Build history of the part. All positions in model axes, mm. Face numbers are marked on the shaded views. Give positions to 0.01 mm unless a question says otherwise; leave off trailing zeros. Order: outer loops, then holes, each group sorted by start corner. A loop starts at its lowest first (then second) coordinate and runs counter-clockwise, first axis right, second up. Notation, with made-up numbers: (53.5, 1.5) - (58.5, 1.5) arc R18 cw to (58.5, 33.5) - close; hole circle Ø1 at (-11.75, -19). An arc over 180 degrees is marked (long way). Write each question's results on one line, items separated by ' | '. Start each with the question number.
1) Cut at A-A on z = 0. List the corners of the cut face in (x, y).
2) Drill centre lines: line 1 along X through (y, z) = (13.6, 0); line 2 along Y through (x, z) = (-67.5, -224.5); line 3 along X through (y, z) = (-13.05, -235). Where is each one in solid material? Low to high. Write a range as from..to.
3) Two-plate mould, pull along X, no slides. Class the marked faces 1, 2 and 3: +X half, -X half, draft (parallel to the pull), parting line (faces both ways), or undercut.
4) Cut at D-D on z = 145.5. List the corners of the cut face in (x, y).
5) Drop flat-ended pins along their axis: pin 1 Ø14 at (x, z) = (-203.52, 117.5) entering from +Y; pin 2 Ø6 at (y, z) = (13, -211) entering from -X; pin 3 Ø5 at (x, y) = (-31, 8.5) entering from -Z. Give the stop position or say it passes through.
6) Cut at C-C on x = 74.5. List the corners of the cut face in (y, z).
7) Cut at B-B on x = -235. List the corners of the cut face in (y, z).
from build123d import *

# Parameters (mm, degrees)
SKETCH1_R           = 260
SKETCH1_R_2         = 6
SKETCH1_R_3         = 219.5
BOSS_EXTRUDE1_DEPTH = 17
SKETCH2_R           = 250
CUT_EXTRUDE1_DEPTH  = 12
CUT_EXTRUDE2_DEPTH  = 370.264133108
BOSS_EXTRUDE2_DEPTH = 130


with BuildPart() as part:
    # Sketch1 → Boss-Extrude1 (new, symmetric)
    with BuildSketch(Plane(origin=(0, 0, 0), x_dir=(1, 0, 0), z_dir=(0, 1, 0))):
        with Locations(Location((0, 0, 0), (0, 0, 270))):
            Circle(SKETCH1_R)
        with Locations(Location((-117.5, 203.515969889, 0), (0, 0, 270))):
            Circle(SKETCH1_R_2, mode=Mode.SUBTRACT)
        with Locations(Location((-203.515969889, 117.5, 0), (0, 0, 270))):
            Circle(SKETCH1_R_2, mode=Mode.SUBTRACT)
        with Locations(Location((-235, 0, 0), (0, 0, 270))):
            Circle(SKETCH1_R_2, mode=Mode.SUBTRACT)
        with Locations(Location((-203.515969889, -117.5, 0), (0, 0, 270))):
            Circle(SKETCH1_R_2, mode=Mode.SUBTRACT)
        with Locations(Location((-117.5, -203.515969889, 0), (0, 0, 270))):
            Circle(SKETCH1_R_2, mode=Mode.SUBTRACT)
        with Locations(Location((0, -235, 0), (0, 0, 270))):
            Circle(SKETCH1_R_2, mode=Mode.SUBTRACT)
        with Locations(Location((117.5, -203.515969889, 0), (0, 0, 270))):
            Circle(SKETCH1_R_2, mode=Mode.SUBTRACT)
        with Locations(Location((203.515969889, -117.5, 0), (0, 0, 270))):
            Circle(SKETCH1_R_2, mode=Mode.SUBTRACT)
        with Locations(Location((235, 0, 0), (0, 0, 270))):
            Circle(SKETCH1_R_2, mode=Mode.SUBTRACT)
        with Locations(Location((203.515969889, 117.5, 0), (0, 0, 270))):
            Circle(SKETCH1_R_2, mode=Mode.SUBTRACT)
        with Locations(Location((117.5, 203.515969889, 0), (0, 0, 270))):
            Circle(SKETCH1_R_2, mode=Mode.SUBTRACT)
        with Locations(Location((0, 235, 0), (0, 0, 270))):
            Circle(SKETCH1_R_2, mode=Mode.SUBTRACT)
        with Locations(Location((0, 0, 0), (0, 0, 270))):
            Circle(SKETCH1_R_3, mode=Mode.SUBTRACT)
    extrude(amount=BOSS_EXTRUDE1_DEPTH, both=True)

    # Sketch2 → Cut-Extrude1 (cut, symmetric)
    with BuildSketch(Plane(origin=(0, 0, 0), x_dir=(1, 0, 0), z_dir=(0, 1, 0))):
        with Locations(Location((0, 0, 0), (0, 0, 270))):
            Circle(SKETCH2_R)
    extrude(amount=CUT_EXTRUDE1_DEPTH, both=True, mode=Mode.SUBTRACT)

    # Sketch3 → Cut-Extrude2 (cut, through all)
    with BuildSketch(Plane(origin=(0, 17, 0), x_dir=(1, 0, 0), z_dir=(0, 1, 0))):
        Polygon((-183.847763109, -183.847763109), (183.847763109, 183.847763109), (370.704407613, -3.008881396), (3.008881396, -370.704407613), align=None)
    extrude(amount=-CUT_EXTRUDE2_DEPTH, mode=Mode.SUBTRACT)

    # Sketch4 → Boss-Extrude2 (add)
    with BuildSketch(Plane(origin=(0, 17, 0), x_dir=(1, 0, 0), z_dir=(0, 1, 0))):
        Polygon((-215.771524586, 145.060846467), (-190.56527753, 119.854599411), (-119.854599411, 190.56527753), (-145.060846467, 215.771524586), align=None)
    extrude(amount=BOSS_EXTRUDE2_DEPTH)


solid = part.part
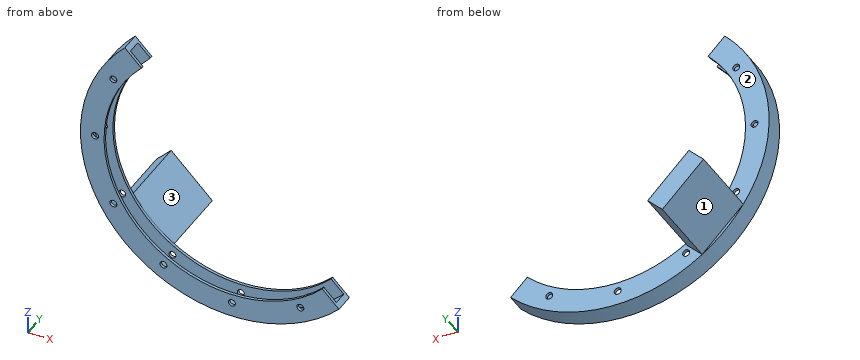
Results:
1) outline: (-260, -17) - (-241, -17) - (-241, -12) - (-250, -12) - (-250, 12) - (-241, 12) - (-241, 17) - (-260, 17) - close; (-229, -17) - (-219.5, -17) - (-219.5, -12) - (-229, -12) - close; (-229, 12) - (-219.5, 12) - (-219.5, 17) - (-229, 17) - close
2) line 1: -260..-241, -229..-219.5 | line 2: -17..-12, 12..17 | line 3: -111.24..-6, 6..111.24
3) face 1: -X half | face 2: draft | face 3: +X half
4) outline: (-215.48, -17) - (-164.35, -17) - (-164.35, -12) - (-203.3, -12) - (-203.3, 12) - (-164.35, 12) - (-164.35, 17) - (-215.48, 17) - close
5) pin 1: y = 17 | pin 2: x = -156 | pin 3: z = -258.43
6) outline: (-17, -249.1) - (17, -249.1) - (17, -206.47) - (12, -206.47) - (12, -238.64) - (-12, -238.64) - (-12, -206.47) - (-17, -206.47) - close
7) outline: (-17, -111.24) - (17, -111.24) - (17, -6) - (12, -6) - (12, -85.29) - (-12, -85.29) - (-12, -6) - (-17, -6) - close; (-17, 6) - (-12, 6) - (-12, 85.29) - (12, 85.29) - (12, 6) - (17, 6) - (17, 111.24) - (-17, 111.24) - close
